from build123d import *

# Parameters (mm, degrees)
SKETCH1_R           = 18
SKETCH1_R_2         = 2
SKETCH1_W           = 10.25
SKETCH1_H           = 10.25
BOSS_EXTRUDE1_DEPTH = 57
CUT_EXTRUDE1_START  = -7
CUT_EXTRUDE1_DEPTH  = 7
SKETCH4_W           = 9.35
SKETCH4_H           = 9.35
CUT_EXTRUDE3_DEPTH  = 20.4
CUT_EXTRUDE4_START  = -40
CUT_EXTRUDE4_DEPTH  = 40
SKETCH6_R           = 1.5
CUT_EXTRUDE5_DEPTH  = 70.267597042
SKETCH7_R           = 3
CUT_EXTRUDE6_DEPTH  = 3
CUT_EXTRUDE7_DEPTH  = 4
CHAMFER1_SIZE       = 1
CHAMFER1_SIZE_2     = 2.747477419
CUT_EXTRUDE8_DEPTH  = 63.42595614
SKETCH12_R          = 1.4
CUT_EXTRUDE10_DEPTH = 20
SKETCH13_R          = 20
SKETCH13_R_2        = 1.4
BOSS_EXTRUDE2_DEPTH = 3
BOSS_EXTRUDE3_DEPTH = 3


with BuildPart() as part:
    # Sketch1 → Boss-Extrude1 (new body)
    with BuildSketch(Plane(origin=(0, 0, 0), x_dir=(1, 0, 0), z_dir=(0, 1, 0))):
        with Locations(Location((0, 0, 0), (0, 0, 90))):
            Circle(SKETCH1_R)
        with Locations(Location((-12, 0, 0), (0, 0, 90))):
            Circle(SKETCH1_R_2, mode=Mode.SUBTRACT)
        Rectangle(SKETCH1_W, SKETCH1_H, mode=Mode.SUBTRACT)
    extrude(amount=BOSS_EXTRUDE1_DEPTH)

    # Sketch2 → Cut-Extrude1 (cut)
    with BuildSketch(Plane(origin=(0, 57, 0), x_dir=(1, 0, 0), z_dir=(0, 1, 0)).offset(CUT_EXTRUDE1_START)):
        with BuildLine():
            Line((-10.8, 5), (-17.291616466, 5))
            ThreePointArc((-17.291616466, 5), (-18, 0), (-17.291616466, -5))
            Line((-17.291616466, -5), (-10.8, -5))
            ThreePointArc((-10.8, -5), (-5.8, 0), (-10.8, 5))
        make_face()
    extrude(amount=CUT_EXTRUDE1_DEPTH, mode=Mode.SUBTRACT)

    # Sketch4 → Cut-Extrude3 (cut)
    with BuildSketch(Plane(origin=(0, 0, 0), x_dir=(-1, 0, 0), z_dir=(0, -1, 0))):
        with Locations((11.135393506, 0.872889968)):
            Rectangle(SKETCH4_W, SKETCH4_H)
    extrude(amount=-CUT_EXTRUDE3_DEPTH, mode=Mode.SUBTRACT)

    # Sketch5 → Cut-Extrude4 (cut)
    with BuildSketch(Plane(origin=(0, 57, 0), x_dir=(1, 0, 0), z_dir=(0, 1, 0)).offset(CUT_EXTRUDE4_START)):
        with BuildLine():
            Line((5.916079783, 17), (-5.916079783, 17))
            ThreePointArc((-5.916079783, 17), (0, 18), (5.916079783, 17))
        make_face()
        with BuildLine():
            Line((5.916079783, -17), (-5.916079783, -17))
            ThreePointArc((-5.916079783, -17), (0, -18), (5.916079783, -17))
        make_face()
    extrude(amount=CUT_EXTRUDE4_DEPTH, mode=Mode.SUBTRACT)

    # Sketch6 → Cut-Extrude5 (cut, through all)
    with BuildSketch(Plane(origin=(0, 0, -17), x_dir=(-1, 0, 0), z_dir=(0, 0, -1))):
        with Locations((0, 47)):
            Circle(SKETCH6_R)
        with Locations((0, 22)):
            Circle(SKETCH6_R)
    extrude(amount=-CUT_EXTRUDE5_DEPTH, mode=Mode.SUBTRACT)

    # Sketch7 → Cut-Extrude6 (cut)
    with BuildSketch(Plane(origin=(0, 0, -17), x_dir=(-1, 0, 0), z_dir=(0, 0, -1))):
        with Locations((0, 47)):
            Circle(SKETCH7_R)
        with Locations((0, 22)):
            Circle(SKETCH7_R)
    extrude(amount=-CUT_EXTRUDE6_DEPTH, mode=Mode.SUBTRACT)

    # Sketch8 → Cut-Extrude7 (cut)
    with BuildSketch(Plane.XY.offset(17)):
        Polygon((0, 43.8), (2.771281292, 45.4), (2.771281292, 48.6), (0, 50.2), (-2.771281292, 48.6), (-2.771281292, 45.4), align=None)
        Polygon((0, 18.8), (2.771281292, 20.4), (2.771281292, 23.6), (0, 25.2), (-2.771281292, 23.6), (-2.771281292, 20.4), align=None)
    extrude(amount=-CUT_EXTRUDE7_DEPTH, mode=Mode.SUBTRACT)

    # Chamfer1
    # the kernel refuses this chamfer: 2.747477419, 1 mm, written as the material it takes off along each edge
    with BuildSketch(Plane(origin=(-5.125, 57, -5.125), x_dir=(0, 0.09904090225204956, -0.9950833631817488), z_dir=(1, 0, 0)), Plane(origin=(-5.125, 57, 5.125), x_dir=(-0.9950833631817488, 0.09904090225204956, 0), z_dir=(0, 0, -1)), Plane(origin=(5.125, 57, 5.125), x_dir=(0, 0.09904090225204956, 0.9950833631817488), z_dir=(-1, 0, 0)), Plane(origin=(5.125, 57, -5.125), x_dir=(0.9950833631817488, 0.09904090225204956, 0), z_dir=(0, 0, 1))) as chamfer1_piece_1:
        Polygon((CHAMFER1_SIZE * 0.995083363182, -CHAMFER1_SIZE * 0.099040902252), (-CHAMFER1_SIZE_2 * 0.0990409022684, -CHAMFER1_SIZE_2 * 0.995083363346), (0, 0), align=None)
    extrude(amount=10.25, mode=Mode.SUBTRACT)
    with BuildSketch(Plane(origin=(-5.125, 57, 5.125), x_dir=(-0.9950833631817488, 0.09904090225204956, 0), z_dir=(0, 0, -1))) as chamfer1_piece_2a_section:
        Polygon((CHAMFER1_SIZE * 0.995083363182, -CHAMFER1_SIZE * 0.099040902252), (-CHAMFER1_SIZE_2 * 0.0990409022684, -CHAMFER1_SIZE_2 * 0.995083363346), (0, 0), align=None)
    chamfer1_piece_2a = extrude(amount=17.377491449, mode=Mode.PRIVATE)
    chamfer1_piece_2a = split(chamfer1_piece_2a, bisect_by=Plane(origin=(-5.432505006, 56.059901151, -5.125), z_dir=(0, 0, -1)), keep=Keep.TOP, mode=Mode.PRIVATE)
    with BuildSketch(Plane(origin=(-12.252491449, 57, -5.125), x_dir=(0, 0.09904090225204956, -0.9950833631817488), z_dir=(1, 0, 0))) as chamfer1_piece_2b_section:
        Polygon((CHAMFER1_SIZE * 0.995083363182, -CHAMFER1_SIZE * 0.099040902252), (-CHAMFER1_SIZE_2 * 0.0990409022684, -CHAMFER1_SIZE_2 * 0.995083363346), (0, 0), align=None)
    chamfer1_piece_2b = extrude(amount=17.377491449, mode=Mode.PRIVATE)
    chamfer1_piece_2b = split(chamfer1_piece_2b, bisect_by=Plane(origin=(-5.125, 56.059901151, -5.432505006), z_dir=(-1, 0, 0)), keep=Keep.TOP, mode=Mode.PRIVATE)
    chamfer1_piece_2 = chamfer1_piece_2a & chamfer1_piece_2b
    add(chamfer1_piece_2, mode=Mode.SUBTRACT)
    with BuildSketch(Plane(origin=(5.125, 57, -12.252491449), x_dir=(0.9950833631817488, 0.09904090225204956, 0), z_dir=(0, 0, 1))) as chamfer1_piece_3a_section:
        Polygon((CHAMFER1_SIZE * 0.995083363182, -CHAMFER1_SIZE * 0.099040902252), (-CHAMFER1_SIZE_2 * 0.0990409022684, -CHAMFER1_SIZE_2 * 0.995083363346), (0, 0), align=None)
    chamfer1_piece_3a = extrude(amount=17.377491449, mode=Mode.PRIVATE)
    chamfer1_piece_3a = split(chamfer1_piece_3a, bisect_by=Plane(origin=(5.432505006, 56.059901151, -5.125), z_dir=(0, 0, -1)), keep=Keep.TOP, mode=Mode.PRIVATE)
    with BuildSketch(Plane(origin=(-5.125, 57, -5.125), x_dir=(0, 0.09904090225204956, -0.9950833631817488), z_dir=(1, 0, 0))) as chamfer1_piece_3b_section:
        Polygon((CHAMFER1_SIZE * 0.995083363182, -CHAMFER1_SIZE * 0.099040902252), (-CHAMFER1_SIZE_2 * 0.0990409022684, -CHAMFER1_SIZE_2 * 0.995083363346), (0, 0), align=None)
    chamfer1_piece_3b = extrude(amount=17.377491449, mode=Mode.PRIVATE)
    chamfer1_piece_3b = split(chamfer1_piece_3b, bisect_by=Plane(origin=(5.125, 56.059901151, -5.432505006), z_dir=(1, 0, 0)), keep=Keep.TOP, mode=Mode.PRIVATE)
    chamfer1_piece_3 = chamfer1_piece_3a & chamfer1_piece_3b
    add(chamfer1_piece_3, mode=Mode.SUBTRACT)
    with BuildSketch(Plane(origin=(5.125, 57, 5.125), x_dir=(0, 0.09904090225204956, 0.9950833631817488), z_dir=(-1, 0, 0))) as chamfer1_piece_4a_section:
        Polygon((CHAMFER1_SIZE * 0.995083363182, -CHAMFER1_SIZE * 0.099040902252), (-CHAMFER1_SIZE_2 * 0.0990409022684, -CHAMFER1_SIZE_2 * 0.995083363346), (0, 0), align=None)
    chamfer1_piece_4a = extrude(amount=17.377491449, mode=Mode.PRIVATE)
    chamfer1_piece_4a = split(chamfer1_piece_4a, bisect_by=Plane(origin=(-5.125, 56.059901151, 5.432505006), z_dir=(-1, 0, 0)), keep=Keep.TOP, mode=Mode.PRIVATE)
    with BuildSketch(Plane(origin=(-5.125, 57, 12.252491449), x_dir=(-0.9950833631817488, 0.09904090225204956, 0), z_dir=(0, 0, -1))) as chamfer1_piece_4b_section:
        Polygon((CHAMFER1_SIZE * 0.995083363182, -CHAMFER1_SIZE * 0.099040902252), (-CHAMFER1_SIZE_2 * 0.0990409022684, -CHAMFER1_SIZE_2 * 0.995083363346), (0, 0), align=None)
    chamfer1_piece_4b = extrude(amount=17.377491449, mode=Mode.PRIVATE)
    chamfer1_piece_4b = split(chamfer1_piece_4b, bisect_by=Plane(origin=(-5.432505006, 56.059901151, 5.125), z_dir=(0, 0, 1)), keep=Keep.TOP, mode=Mode.PRIVATE)
    chamfer1_piece_4 = chamfer1_piece_4a & chamfer1_piece_4b
    add(chamfer1_piece_4, mode=Mode.SUBTRACT)
    with BuildSketch(Plane(origin=(12.252491449, 57, 5.125), x_dir=(0, 0.09904090225204956, 0.9950833631817488), z_dir=(-1, 0, 0))) as chamfer1_piece_5a_section:
        Polygon((CHAMFER1_SIZE * 0.995083363182, -CHAMFER1_SIZE * 0.099040902252), (-CHAMFER1_SIZE_2 * 0.0990409022684, -CHAMFER1_SIZE_2 * 0.995083363346), (0, 0), align=None)
    chamfer1_piece_5a = extrude(amount=17.377491449, mode=Mode.PRIVATE)
    chamfer1_piece_5a = split(chamfer1_piece_5a, bisect_by=Plane(origin=(5.125, 56.059901151, 5.432505006), z_dir=(1, 0, 0)), keep=Keep.TOP, mode=Mode.PRIVATE)
    with BuildSketch(Plane(origin=(5.125, 57, -5.125), x_dir=(0.9950833631817488, 0.09904090225204956, 0), z_dir=(0, 0, 1))) as chamfer1_piece_5b_section:
        Polygon((CHAMFER1_SIZE * 0.995083363182, -CHAMFER1_SIZE * 0.099040902252), (-CHAMFER1_SIZE_2 * 0.0990409022684, -CHAMFER1_SIZE_2 * 0.995083363346), (0, 0), align=None)
    chamfer1_piece_5b = extrude(amount=17.377491449, mode=Mode.PRIVATE)
    chamfer1_piece_5b = split(chamfer1_piece_5b, bisect_by=Plane(origin=(5.432505006, 56.059901151, 5.125), z_dir=(0, 0, 1)), keep=Keep.TOP, mode=Mode.PRIVATE)
    chamfer1_piece_5 = chamfer1_piece_5a & chamfer1_piece_5b
    add(chamfer1_piece_5, mode=Mode.SUBTRACT)

    # Sketch9 → Cut-Extrude8 (cut, through all)
    with BuildSketch(Plane.XZ):
        with BuildLine():
            Line((-7.454203172, -7.297889968), (-15.454203172, -7.297889968))
            ThreePointArc((-15.454203172, -7.297889968), (-13.761984914, -9.955415688), (-11.632322635, -12.277178848))
            Line((-11.632322635, -12.277178848), (-7.454203172, -7.297889968))
        make_face()
    extrude(amount=-CUT_EXTRUDE8_DEPTH, mode=Mode.SUBTRACT)

    # Sketch12 → Cut-Extrude10 (cut)
    with BuildSketch(Plane(origin=(0, 57, 0), x_dir=(1, 0, 0), z_dir=(0, 1, 0))):
        with Locations(Location((10, 0, 0), (0, 0, 270))):
            Circle(SKETCH12_R)
        with Locations(Location((-9.192388155, -9.192388155, 0), (0, 0, 270))):
            Circle(SKETCH12_R)
    extrude(amount=-CUT_EXTRUDE10_DEPTH, mode=Mode.SUBTRACT)

    # Sketch13 → Boss-Extrude2 (add)
    with BuildSketch(Plane(origin=(0, 57, 0), x_dir=(1, 0, 0), z_dir=(0, 1, 0))):
        with Locations(Location((0, 0, 0), (0, 0, 270))):
            Circle(SKETCH13_R)
        with Locations(Location((10, 0, 0), (0, 0, 270))):
            Circle(SKETCH13_R_2, mode=Mode.SUBTRACT)
        with Locations(Location((-9.192388155, -9.192388155, 0), (0, 0, 270))):
            Circle(SKETCH13_R_2, mode=Mode.SUBTRACT)
        with BuildLine():
            Line((-10.8, 5), (-17.291616466, 5))
            Line((-17.291616466, 5), (-17.291616466, -5))
            Line((-17.291616466, -5), (-10.8, -5))
            ThreePointArc((-10.8, -5), (-7.959770503, -4.114984375), (-6.125, -1.773238563))
            Line((-6.125, -1.773238563), (-6.125, -6.125))
            Line((-6.125, -6.125), (6.125, -6.125))
            Line((6.125, -6.125), (6.125, 6.125))
            Line((6.125, 6.125), (-6.125, 6.125))
            Line((-6.125, 6.125), (-6.125, 1.773238563))
            ThreePointArc((-6.125, 1.773238563), (-7.959770503, 4.114984375), (-10.8, 5))
        make_face(mode=Mode.SUBTRACT)
        with BuildLine():
            Line((-7.454203172, 7.297889968), (-15.454203172, 7.297889968))
            ThreePointArc((-15.454203172, 7.297889968), (-13.761984914, 9.955415688), (-11.632322635, 12.277178848))
            Line((-11.632322635, 12.277178848), (-7.454203172, 7.297889968))
        make_face(mode=Mode.SUBTRACT)
    extrude(amount=BOSS_EXTRUDE2_DEPTH)

    # Sketch14 → Boss-Extrude3 (add)
    with BuildSketch(Plane(origin=(0, 60, 0), x_dir=(1, 0, 0), z_dir=(0, 1, 0))):
        with BuildLine():
            Line((12.855752194, 15.320888862), (14.321646009, 13.960317173))
            ThreePointArc((14.321646009, 13.960317173), (14.268984946, 15.373549926), (12.855752194, 15.320888862))
        make_face()
    extrude(amount=-BOSS_EXTRUDE3_DEPTH)


solid = part.part
Here's how the part is built. I have some questions about the finished solid (model axes, mm). A direction names the side the tool comes from. Round coordinates to 2 decimals unless told otherwise and drop trailing zeros. Write each loop counter-clockwise with the first axis right and the second up, starting at its lowest first coordinate (ties: lowest second). Pieces come first, ordered by that corner, then holes.
1. Suppose I cut it at A-A (y = 22). List the corners of the cut face in (x, z) for me (3 decimals).
2. Suppose I cut it at C-C (y = 36). List the corners of the cut face in (x, z) for me (3 decimals).
3. If we mould it in two halves opening along Y, with no side actions, what happens to faces 4 (the flat face through (-14, 55, 5)), 5 (the flat face through (-1.405, 44.611, 15.028)), 6 (the cylindrical face through (0.325, 45.536, 9.007)), 7 (the flat face through (5.632, 55.645, -0.086))? For each: released by +Y, released by -Y, zero draft, split by the parting line, or undercut.
4. Suppose I cut it at B-B (z = -11). List the corners of the cut face in (x, y) for me, and give its area (3 significant figures).
5. Will these pins go through, and if not, where does the flat tip stop? pin 1 Ø8 at (x, y) = (0.5, 33) entering from -Z; pin 2 Ø8 at (x, y) = (-7, 37) entering from +Z; pin 3 Ø3 at (x, y) = (-11, 11.5) entering from -Z; pin 4 Ø2 at (x, z) = (-15.5, -14.5) entering from +Y.
6. Suppose I cut it at D-D (z = 0). State how many separate pieces and enclosed holes the cut face has, and give its area (3 significant figures).
7. I need wall thicknesses on L1, parallel to Y at x = 0, z = 11; L2, parallel to Y at x = 0, z = -15; L3, parallel to X at y = 46.75, z = 0 (3 decimals). Which ranges of each line are inside material? Lowest first, please.
8. For faces 1 (the flat face through (-15.81, 10, -1)), 2 (the flat face through (5.125, 27, 0)), 3 (the flat face through (-17.292, 58, 0)), which set-ups out of +Z, -Z, +X, -X, +Y, -Y let a thin tool reach every point of the face, with its end or its side?
Answer sheet:
1. outline: (-5.916, -17) - (-3, -17) - (-3, -14) - (-1.5, -14) - (-1.5, -5.125) - (-5.125, -5.125) - (-5.125, 5.125) - (-1.5, 5.125) - (-1.5, 13) - (-2.771, 13) - (-2.771, 17) - (-5.916, 17) arc R18 ccw to start; (1.5, -14) - (3, -14) - (3, -17) - (5.916, -17) arc R18 ccw to (5.916, 17) - (2.771, 17) - (2.771, 13) - (1.5, 13) - (1.5, 5.125) - (5.125, 5.125) - (5.125, -5.125) - (1.5, -5.125) - close; hole (-15.454, -7.298) arc R18 ccw to (-11.632, -12.277) - (-7.454, -7.298) - close; hole circle Ø4 at (-12, 0)
2. outline: (-5.916, -17) - (5.916, -17) arc R18 ccw to (5.916, 17) - (-5.916, 17) arc R18 ccw to start; hole (-15.454, -7.298) arc R18 ccw to (-11.632, -12.277) - (-7.454, -7.298) - close; hole circle Ø4 at (-12, 0); hole (-5.125, -5.125) - (5.125, -5.125) - (5.125, 5.125) - (-5.125, 5.125) - close
3. face 4: zero draft
3. face 5: undercut
3. face 6: undercut
3. face 7: released by +Y
4. outline: (-16.7, 57) - (-14.25, 57) - (-14.25, 0) - (-12.9, 0) - (-12.9, 60) - (-16.7, 60) - close; (-10.56, 0) - (14.25, 0) - (14.25, 57) - (16.7, 57) - (16.7, 60) - (-10.56, 60) - close; hole circle Ø3 at (0, 22); hole circle Ø3 at (0, 47)
4. area: 1,570 mm2
5. pin 1: stops at z = -17
5. pin 2: stops at z = 17
5. pin 3: stops at z = -15.29
5. pin 4: passes through
6. separate pieces: 4
6. enclosed holes: 0
6. area: 1,060 mm2
7. L1: y = 0 to 20.5, 23.5 to 45.5, 48.5 to 60
7. L2: y = 0 to 19, 25 to 44, 50 to 60
7. L3: x = -18 to -14, -10 to -5.125, 5.125 to 8.6, 11.4 to 18
8. face 1: -Y
8. face 2: +Y, -Y
8. face 3: +Y
